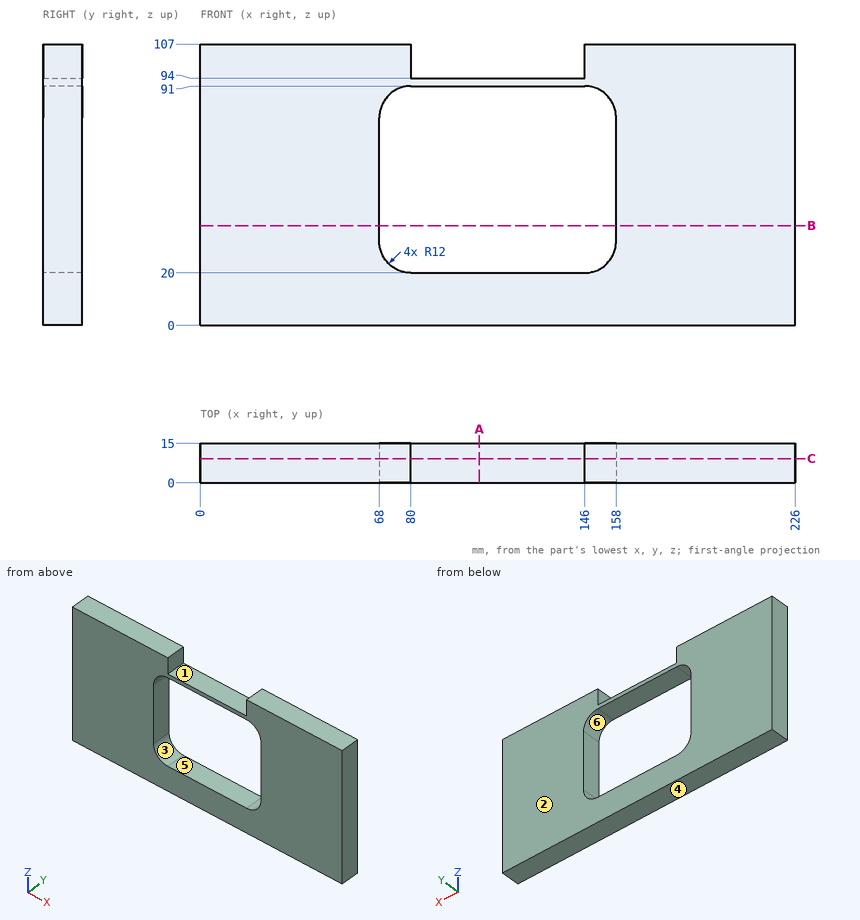
Part print with two shaded views. Sizes in mm from the minimum x, y, z corner. A direction names the side the tool comes from. Coordinates: 2 decimals unless noted, no trailing zeros. Loops run counter-clockwise (first coordinate to the right, second up) from the corner with the lowest first, then second, coordinate; pieces in that order, holes last. Notation, with made-up numbers: M 49.5,-21 L 55.5,-21 A4 cw 55.5,-14 Z; hole C -33.5,-16.75 d7. An arc over 180 degrees is marked long. Use CSV: the item, a comma, the result in double quotes. Start each with the question number.
1. Band-saw the part on C-C, the plane y = 9.25. List the corners of the cut face in (x, z).
2. Probe probe 1 along X at (y, z) = (7, 75); probe 2 along Z at (x, y) = (106.5, 12.75); probe 3 along X at (y, z) = (5, 30.5). List the from-to ranges inside material, lowest first. Write a range as [from, to].
3. Band-saw the part on A-A, the plane x = 106. List the corners of the cut face in (y, z), then the cut area to 3 significant figures.
4. Flat gauge pins, fed straight in: pin 1 (4.5 mm diameter, centred on x = 124.5, y = 7, fed in from +Z); pin 2 (5 mm diameter, centred on x = 73.5, z = 28, fed in from +Y). Where does each tip first touch, or does it go through?
5. Tool access for the marked faces 1, 2 and 3: list every direction of +Z, -Z, +X, -X, +Y, -Y with a clear straight run to the whole face (end or side of a thin tool).
6. Band-saw the part on B-B, the plane z = 38. List the corners of the cut face in (x, y), then the cut area to 3 significant figures.
7. Two-plate mould, pull along X, no slides. Class the marked faces 4, 5 and 6: pulls with the +X half, pulls with the -X half, needs draft (parallel to the pull), parting line crosses it, or undercut.
Entries:
1,outline,"M 0,0 L 226,0 L 226,107 L 146,107 L 146,94 L 80,94 L 80,107 L 0,107 Z; hole M 68,32 A12 ccw 80,20 L 146,20 A12 ccw 158,32 L 158,79 A12 ccw 146,91 L 80,91 A12 ccw 68,79 Z"
2,probe 1,"x = [0, 68], [158, 226]"
2,probe 2,"z = [0, 20], [91, 94]"
2,probe 3,"x = [0, 68.09], [157.91, 226]"
3,outline,"M 0,0 L 15,0 L 15,20 L 0,20 Z; M 0,91 L 15,91 L 15,94 L 0,94 Z"
3,area,"345 mm2"
4,pin 1,"stops at z = 94"
4,pin 2,"passes through"
5,face 1,"+Z, +Y, -Y"
5,face 2,"+Z, -Z, +X, -X, +Y"
5,face 3,"+Y, -Y"
6,outline,"M 0,0 L 68,0 L 68,15 L 0,15 Z; M 158,0 L 226,0 L 226,15 L 158,15 Z"
6,area,"2,040 mm2"
7,face 4,"needs draft"
7,face 5,"undercut"
7,face 6,"undercut"
